from build123d import *

# Parameters (mm, degrees)
F1_DEPTH = 119.822524
F2_R     = 34.250378
F3_T     = -5
F4_R     = 25
F5_DEPTH = 25


with BuildPart() as f1:
    # F0 (on Top) → F1 (new body, symmetric)
    with BuildSketch(Plane.XY):
        Polygon((-76.817763, -68.995313), (73.182237, -68.995313), (73.182237, 81.004687), (-1.817763, 81.004687), (-76.817763, 81.004687), align=None)
    extrude(amount=F1_DEPTH, both=True)

    # F2
    f2_edges = [f1.edges().sort_by_distance(p)[0] for p in [
        (73.182237, 81.004687, 0),
        (-76.817763, 81.004687, 0),
    ]]
    fillet(f2_edges, radius=F2_R)

    # F3
    f3_openings = [f1.faces().sort_by_distance(p)[0] for p in [
        (-1.817763, 4.463075, 119.822524),
    ]]
    offset(amount=F3_T, openings=f3_openings)

    # F4 (on face) → F5 (cut)
    with BuildSketch(Plane.XZ.offset(68.995313)):
        with Locations((0, 69.822524)):
            Circle(F4_R)
    extrude(amount=-F5_DEPTH, mode=Mode.SUBTRACT)


solid = f1.part
Source: CAD feature listing. Evaluate the final solid. Frame: model axes, mm. A direction names the side the tool comes from. Coordinates: 2 decimals unless noted, no trailing zeros. Loops run counter-clockwise (first coordinate to the right, second up) from the corner with the lowest first, then second, coordinate; pieces in that order, holes last. Notation, with made-up numbers: (17, 1) -> (71, 1) arc R20 ccw to (71, 27) -> close; hole circle Ø11 at (39, -8.75). An arc over 180 degrees is marked (long way). Answer in a Markdown table with one row per item. Add a question column.
Q1. Section B-B on x = 0. Return the cut outline in (y, z).
Q2. Contact query for flat-ended pins moving along their axis: pin 1 Ø4 at (x, z) = (-62, -33.5) entering from +Y; pin 2 Ø5 at (x, y) = (-5.5, 64.5) entering from +Z. Output: stop coordinate, or through.
Q3. Pull-direction query (Y, two-part tool) for faces 3 (the face through (59.39, 67.66, 4.14)), 4 (the face through (62.88, 71.24, 1.68)), 5 (the face through (-5.42, -66.53, 45.417)); classes: pulls with the +Y half, pulls with the -Y half, needs draft (parallel to the pull), parting line crosses it, or undercut.
Q4. Section C-C on y = 50. Return the cut outline in (x, z), and give its area (3 significant figures).
Q5. Section A-A on z = -16.5. Return the cut outline in (x, y).
Q6. Section D-D on x = 53. Return the cut outline in (y, z), and give its area (3 significant figures).
Q7. Reachability of faces 1 (the face through (-2, -66, 119.823)), 2 (the face through (-1, 76.005, 4)) from +Z, -Z, +X, -X, +Y, -Y: full face, straight path, thin tool, end or side. Return the list, or none.
Q8. Ray query, line 1 along X through (y, z) = (32.5, 22); line 2 along Z through (x, y) = (0, -67); line 3 along Y through (x, z) = (-17, 47). Return the intervals inside material, ascending.
Computed values:
| question | item | result |
|---|---|---|
| 1 | outline | (-69, -119.82) -> (81, -119.82) -> (81, 119.82) -> (76, 119.82) -> (76, -114.82) -> (-64, -114.82) -> (-64, 44.82) -> (-69, 44.82) -> close; (-69, 94.82) -> (-64, 94.82) -> (-64, 119.82) -> (-69, 119.82) -> close |
| 2 | pin 1 | stops at y = 76.24 |
| 2 | pin 2 | stops at z = -114.82 |
| 3 | face 3 | undercut |
| 3 | face 4 | pulls with the +Y half |
| 3 | face 5 | needs draft |
| 4 | outline | (-76.66, -119.82) -> (73.03, -119.82) -> (73.03, 119.82) -> (68, 119.82) -> (68, -114.82) -> (-71.64, -114.82) -> (-71.64, 119.82) -> (-76.66, 119.82) -> close |
| 4 | area | 3,110 mm^2 |
| 5 | outline | (-76.82, -69) -> (73.18, -69) -> (73.18, 46.75) arc R34.25 ccw to (38.93, 81) -> (-42.57, 81) arc R34.25 ccw to (-76.82, 46.75) -> close; hole (-71.82, -64) -> (68.18, -64) -> (68.18, 46.75) arc R29.25 ccw to (38.93, 76) -> (-42.57, 76) arc R29.25 ccw to (-71.82, 46.75) -> close |
| 6 | outline | (-69, -119.82) -> (77.98, -119.82) -> (77.98, 119.82) -> (72.4, 119.82) -> (72.4, -114.82) -> (-64, -114.82) -> (-64, 119.82) -> (-69, 119.82) -> close |
| 6 | area | 3,220 mm^2 |
| 7 | face 1 | +Z, +X, -X, +Y, -Y |
| 7 | face 2 | +Z |
| 8 | line 1 | x = -76.82 to -71.82, 68.18 to 73.18 |
| 8 | line 2 | z = -119.82 to 44.82, 94.82 to 119.82 |
| 8 | line 3 | y = -69 to -64, 76 to 81 |
